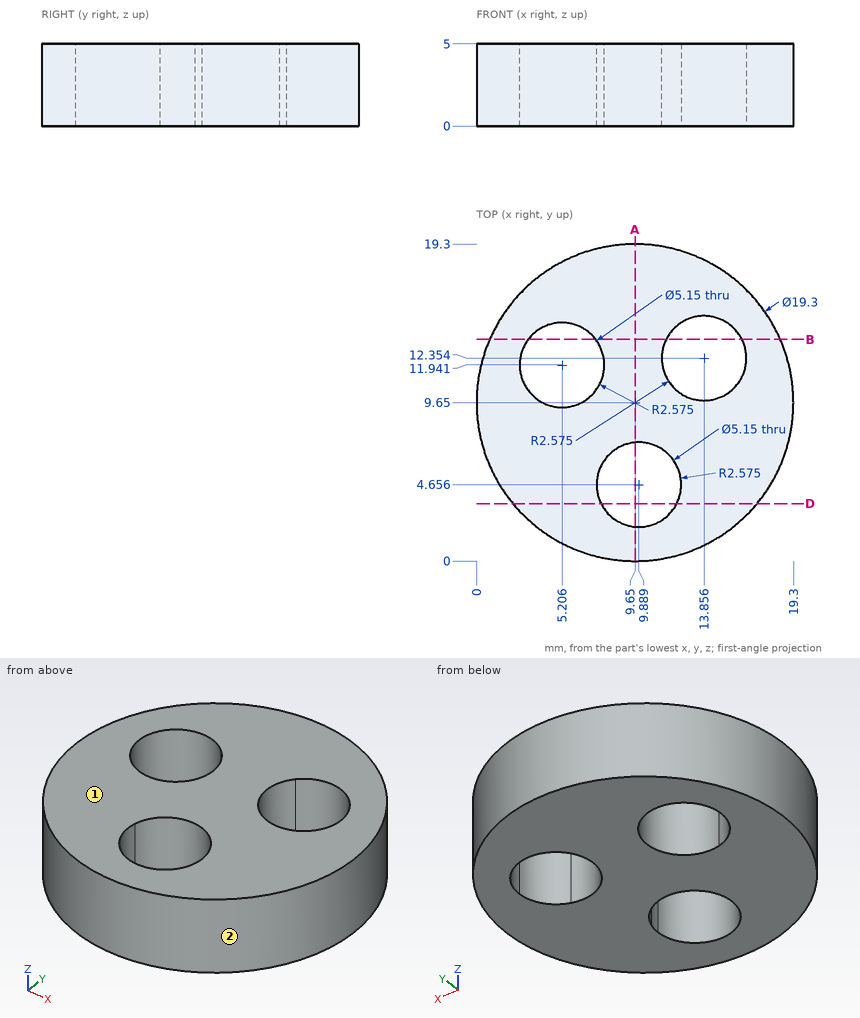
Could you check a few things on this drawing? It's one solid part, dimensions in mm from its lowest x, y, z. Give positions to 0.01 mm unless a question says otherwise; leave off trailing zeros. Order: outer loops, then holes, each group sorted by start corner. A loop starts at its lowest first (then second) coordinate and runs counter-clockwise, first axis right, second up. Notation, with made-up numbers: (6, 50) -> (13, 50) arc R29 cw to (13, 84) -> close; hole circle Ø1 at (23.25, 12.25). An arc over 180 degrees is marked (long way). Answer in a Markdown table with one row per item. Add a question column.
Item 1: Imagine slicing it at D-D (y = 3.5). List the corners of the cut face in (x, z) for me.
Item 2: Imagine slicing it at A-A (x = 9.65). List the corners of the cut face in (y, z) for me.
Item 3: We'd pull the mould along X, two halves only. Please class the marked faces 1 and 2: pulls with the +X half, pulls with the -X half, needs draft (parallel to the pull), parting line crosses it, or undercut.
Item 4: Please list where these lines run through material, in increasing order: probe 1 along X at (y, z) = (10, 0.7) (1 decimal); probe 2 along X at (y, z) = (12.5, 4.15) (1 decimal); probe 3 along Y at (x, z) = (14, 3.3) (1 decimal).
Item 5: Imagine slicing it at B-B (y = 13.5). Count the separate pieces of the cut face and the enclosed holes in it.
Item 6: I'm going to push flat-ended pins straight in: P1, Ø6, axis at x = 4, y = 12.5, coming from the +Z side; P2, Ø4.5, axis at x = 9.89, y = 4.66, coming from the +Z side; P3, Ø1, axis at y = 5, z = 2.5, coming from the -X side; P4, Ø2, axis at x = 16, z = 3, coming from the +Y side. Where does each tip first touch, or does it pass through?
Result:
| question | item | result |
|---|---|---|
| 1 | outline | (2.21, 0) -> (7.59, 0) -> (7.59, 5) -> (2.21, 5) -> close; (12.19, 0) -> (17.09, 0) -> (17.09, 5) -> (12.19, 5) -> close |
| 2 | outline | (0, 0) -> (2.09, 0) -> (2.09, 5) -> (0, 5) -> close; (7.22, 0) -> (19.3, 0) -> (19.3, 5) -> (7.22, 5) -> close |
| 3 | face 1 | needs draft |
| 3 | face 2 | parting line crosses it |
| 4 | probe 1 | 0 to 3.5, 6.9 to 12.8, 14.9 to 19.3 |
| 4 | probe 2 | 0.4 to 2.7, 7.7 to 11.3, 16.4 to 18.9 |
| 4 | probe 3 | 1 to 9.8, 14.9 to 18.3 |
| 5 | separate pieces | 3 |
| 5 | enclosed holes | 0 |
| 6 | P1 | z = 5 |
| 6 | P2 | through |
| 6 | P3 | x = 0.94 |
| 6 | P4 | y = 17.68 |
